```python
from build123d import *

# Parameters (mm, degrees)
SKETCH1_R           = 15.75
SKETCH1_R_2         = 1.5
BOSS_EXTRUDE1_DEPTH = 10
SKETCH2_R           = 7
SKETCH2_R_2         = 2.5
CUT_EXTRUDE1_DEPTH  = 1
CUT_EXTRUDE2_START  = -1
SKETCH3_R           = 7
SKETCH3_R_2         = 2.5
CUT_EXTRUDE2_DEPTH  = 1
FILLET1_R           = 3


with BuildPart() as part:
    # Sketch1 → Boss-Extrude1 (new body)
    with BuildSketch(Plane.XY):
        with Locations((-62.5, -49.913872362)):
            Circle(SKETCH1_R)
        with Locations((-62.5, -49.913872362)):
            Circle(SKETCH1_R_2, mode=Mode.SUBTRACT)
    extrude(amount=BOSS_EXTRUDE1_DEPTH)

    # Sketch2 → Cut-Extrude1 (cut)
    with BuildSketch(Plane.XY.offset(10)):
        with Locations((-62.5, -49.913872362)):
            Circle(SKETCH2_R)
        with Locations((-62.5, -49.913872362)):
            Circle(SKETCH2_R_2, mode=Mode.SUBTRACT)
    extrude(amount=-CUT_EXTRUDE1_DEPTH, mode=Mode.SUBTRACT)

    # Sketch3 → Cut-Extrude2 (cut)
    with BuildSketch(Plane(origin=(0, 0, 0), x_dir=(-1, 0, 0), z_dir=(0, 0, -1)).offset(CUT_EXTRUDE2_START)):
        with Locations(Location((62.5, -49.913872362, 0), (0, 0, 180))):
            Circle(SKETCH3_R)
        with Locations(Location((62.5, -49.913872362, 0), (0, 0, 180))):
            Circle(SKETCH3_R_2, mode=Mode.SUBTRACT)
    extrude(amount=CUT_EXTRUDE2_DEPTH, mode=Mode.SUBTRACT)

    # Fillet1
    fillet1_edges = [part.edges().sort_by_distance(p)[0] for p in [
        (-78.25, -49.913872362, 0),
        (-78.25, -49.913872362, 10),
    ]]
    fillet(fillet1_edges, radius=FILLET1_R)


solid = part.part
```
Verification items for the finished model (mm, model axes). A direction names the side the tool comes from. Give positions to 0.01 mm unless a question says otherwise; leave off trailing zeros. Write each loop counter-clockwise with the first axis right and the second up, starting at its lowest first coordinate (ties: lowest second). Pieces come first, ordered by that corner, then holes. Notation, with made-up numbers: (-14, 49) - (0, 49) arc R18 cw to (0, 80) - close; hole circle Ø4 at (69, 9). An arc over 180 degrees is marked (long way). Put each result on its own line as item: value.
Q1. Section check B-B on z = 8.25. Record the cut outline in (x, y).
Result:
outline: circle Ø30.95 at (-62.5, -49.91); hole circle Ø3 at (-62.5, -49.91)
Q2. Depth check by flat-ended pin: P1, Ø1, axis at y = -45, z = 6, coming from the -X side; P2, Ø2, axis at y = -39.5, z = 1.5, coming from the -X side; P3, Ø2, axis at x = -64, z = 9, coming from the +Y side; P4, Ø2.5, axis at x = -62.5, y = -49.91, coming from the -Z side. Enter the tip coordinate at first touch or a pass-through.
Result:
P1: x = -77.62
P2: x = -74.81
P3: y = -34.4
P4: through
Q3. Scan lines: probe 1 along Y at (x, z) = (-62.5, 6.5); probe 2 along Y at (x, z) = (-62.5, 0.25); probe 3 along X at (y, z) = (-50, 8.75). Record each from-to range of solid material in increasing order. Write a range as from..to.
Result:
probe 1: -65.66..-51.41, -48.41..-34.16
probe 2: -63.86..-56.91, -52.41..-51.41, -48.41..-47.41, -42.91..-35.96
probe 3: -77.69..-64, -61..-47.31
Q4. Mould release check, pull along Y, two halves, no side actions. Record for faces 4 (the face through (-78.235, -49.221, 4.972)), 5 (the face through (-61, -51, 10)), 6 (the face through (-63, -53, 9)): released by +Y, released by -Y, zero draft, split by the parting line, or undercut.
Result:
face 4: split by the parting line
face 5: zero draft
face 6: undercut
Q5. Section check A-A on x = -62.5. Record the cut outline in (y, z), and give its area (3 significant figures).
Result:
outline: (-65.66, 3) arc R3 ccw to (-62.66, 0) - (-56.91, 0) - (-56.91, 1) - (-52.41, 1) - (-52.41, 0) - (-51.41, 0) - (-51.41, 10) - (-52.41, 10) - (-52.41, 9) - (-56.91, 9) - (-56.91, 10) - (-62.66, 10) arc R3 ccw to (-65.66, 7) - close; (-48.41, 0) - (-47.41, 0) - (-47.41, 1) - (-42.91, 1) - (-42.91, 0) - (-37.16, 0) arc R3 ccw to (-34.16, 3) - (-34.16, 7) arc R3 ccw to (-37.16, 10) - (-42.91, 10) - (-42.91, 9) - (-47.41, 9) - (-47.41, 10) - (-48.41, 10) - close
area: 259 mm2
Q6. Set-up check for faces 1 (the face through (-60.19, -48.96, 0.51)), 2 (the face through (-61.156, -47.806, 9.507)), 3 (the face through (-57, -55, 0)): record each of +Z, -Z, +X, -X, +Y, -Y from which the full face is reachable in a straight line by a thin tool's end or side.
Result:
face 1: -Z
face 2: +Z
face 3: -Z, +X, -X, +Y, -Y
